from build123d import *

# Parameters (mm, degrees)
F0_R     = 6.3373
F1_DEPTH = 6.604
F2_R     = 8.89
F3_DEPTH = 3.175
F4_W     = 15.0394464063
F4_H     = 9.4838521599
F5_DEPTH = 25.4
F6_R     = 3.175
F7_DEPTH = 25.4
F8_R     = 5.08
F9_DEPTH = 12.7


with BuildPart() as f1:
    # F0 (on Top) → F1 (new body)
    with BuildSketch(Plane.XY):
        Circle(F0_R)
    extrude(amount=F1_DEPTH)

    # F2 (on face) → F3 (join)
    with BuildSketch(Plane(origin=(0, 0, 0), x_dir=(1, 0, 0), z_dir=(0, 0, -1))):
        Circle(F2_R)
    extrude(amount=F3_DEPTH)

    # F4 (on face) → F5 (join)
    with BuildSketch(Plane(origin=(0, 0, -3.175), x_dir=(1, 0, 0), z_dir=(0, 0, -1))):
        Rectangle(F4_W, F4_H)
    extrude(amount=F5_DEPTH)

    # F6 (on face) → F7 (cut)
    with BuildSketch(Plane.XZ.offset(4.74192608)):
        with Locations((0, -22.9682382196)):
            Circle(F6_R)
    extrude(amount=-F7_DEPTH, mode=Mode.SUBTRACT)

    # F8
    f8_edges = [f1.edges().sort_by_distance(p)[0] for p in [
        (-7.519723, 0, -28.575),
        (7.519723, 0, -28.575),
    ]]
    fillet(f8_edges, radius=F8_R)

    # F9 (add): a face of the model
    f9_faces = [f1.faces().sort_by_distance(p)[0] for p in [
        (0, 0, 6.604),
    ]]
    extrude(f9_faces, amount=F9_DEPTH)


solid = f1.part
Design review of the part built by this model. Coordinates are the model's own, in mm. A direction names the side the tool comes from. Coordinates: 2 decimals unless noted, no trailing zeros. Write each loop counter-clockwise with the first axis right and the second up, starting at its lowest first coordinate (ties: lowest second). Pieces come first, ordered by that corner, then holes. Notation, with made-up numbers: (-11.75, 41) - (-5.75, 41) arc R23 cw to (-5.75, 64) - close; hole circle Ø11 at (-11, -7.75). An arc over 180 degrees is marked (long way). One line per item, written item: value.
1) To check wall thickness, follow probe 1 along Z at (x, y) = (0, 2.75) (3 decimals); probe 2 along Y at (x, z) = (2, -5.5); probe 3 along Z at (x, y) = (2, -6.5) (3 decimals). State the ranges of each line that lie inside material, in increasing order.
Answer sheet:
probe 1: z = -28.575 to -26.143, -19.793 to 19.304
probe 2: y = -4.74 to 4.74
probe 3: z = -3.175 to 0
2) Add section D-D (z = 3.5). State the section outline as (x, y) points, plus the area to 3 significant figures.
Answer sheet:
outline: circle Ø12.67 at (0, 0)
area: 126 mm2
3) For faces 5 (the face through (0, 6, -3.175)), 6 (the face through (0, -6, -3.175)), 7 (the face through (-8, 0, -3.175)), 8 (the face through (8, 0, -3.175)), 9 (the face through (4, 6, 0)), list the 3-axis set-ups (+Z, -Z, +X, -X, +Y, -Y) from which the entire face can be reached by the end or side of a thin tool; tool diameter is ignored.
Answer sheet:
face 5: -Z, +X, -X, +Y
face 6: -Z, +X, -X, -Y
face 7: -Z, -X, +Y, -Y
face 8: -Z, +X, +Y, -Y
face 9: +Z
4) Add section B-B (y = 4.25). State the section outline as (x, z) points (3 decimals), plus the area to 3 significant figures.
Answer sheet:
outline: (-7.808, -3.175) - (-7.52, -3.175) - (-7.52, -23.495) arc R5.08 ccw to (-2.44, -28.575) - (2.44, -28.575) arc R5.08 ccw to (7.52, -23.495) - (7.52, -3.175) - (7.808, -3.175) - (7.808, 0) - (4.701, 0) - (4.701, 19.304) - (-4.701, 19.304) - (-4.701, 0) - (-7.808, 0) - close; hole circle Ø6.35 at (0, -22.968)
area: 570 mm2
5) Insertion check: pin 1 (1.1 mm diameter, centred on x = -8.5, y = 2, fed in from -Z) (3 decimals); pin 2 (4 mm diameter, centred on x = 0, z = -22.97, fed in from +Y); pin 3 (6 mm diameter, centred on x = 7, z = 5.5, fed in from +Y); pin 4 (4 mm diameter, centred on x = -6.5, z = -5.5, fed in from -Y). Each pin has a flat end and moves straight along its axis. Give the tip position at first contact, or say it passes through.
Answer sheet:
pin 1: stops at z = -3.175
pin 2: passes through
pin 3: stops at y = 4.92
pin 4: stops at y = -4.74
6) Add section A-A (x = 0). State the section outline as (y, z) points (3 decimals), plus the area to 3 significant figures.
Answer sheet:
outline: (-8.89, -3.175) - (-4.742, -3.175) - (-4.742, -19.793) - (4.742, -19.793) - (4.742, -3.175) - (8.89, -3.175) - (8.89, 0) - (6.337, 0) - (6.337, 19.304) - (-6.337, 19.304) - (-6.337, 0) - (-8.89, 0) - close; (-4.742, -28.575) - (4.742, -28.575) - (4.742, -26.143) - (-4.742, -26.143) - close
area: 482 mm2
7) Add section C-C (z = -24). State the section outline as (x, y) points, plus the area to 3 significant figures.
Answer sheet:
outline: (-7.49, -4.74) - (-3, -4.74) - (-3, 4.74) - (-7.49, 4.74) - close; (3, -4.74) - (7.49, -4.74) - (7.49, 4.74) - (3, 4.74) - close
area: 85.2 mm2
8) Mouldability with a two-part tool opening along X and no side actions: class faces 1 (the face through (-0.688, -0.066, -26.068)), 2 (the face through (7.52, 0, -13)), 3 (the face through (0, -4.742, -16)), 4 (the face through (-7.52, 0, -13)) as +X half, -X half, draft (parallel to the pull), parting line (faces both ways), or undercut.
Answer sheet:
face 1: undercut
face 2: +X half
face 3: draft
face 4: -X half
